Geometry: final body of the model. Coordinates: model frame, mm. Face numbers are marked on the shaded views. A direction names the side the tool comes from. Give positions to 0.01 mm unless a question says otherwise; leave off trailing zeros. Order: outer loops, then holes, each group sorted by start corner. A loop starts at its lowest first (then second) coordinate and runs counter-clockwise, first axis right, second up. Notation, with made-up numbers: (-2, 30) - (19, 30) arc R31 ccw to (19, 61) - close; hole circle Ø8 at (21.25, 82.5). An arc over 180 degrees is marked (long way). Use one line per item in the form item = value.
from build123d import *

# Parameters (mm, degrees)
SKETCH_1_W      = 42.3
SKETCH_1_H      = 42.3
SKETCH_1_R      = 11
SKETCH_1_R_2    = 1.5
EXTRUDE_1_DEPTH = 4
SKETCH_2_W      = 38
SKETCH_2_H      = 62.3
SKETCH_2_R      = 1.5
EXTRUDE_2_DEPTH = 4
CHAMFER_1_SIZE  = 6


with BuildPart() as part:
    # 스케치1 → 보스-돌출1 (new body)
    with BuildSketch(Plane.XY):
        Rectangle(SKETCH_1_W, SKETCH_1_H)
        Circle(SKETCH_1_R, mode=Mode.SUBTRACT)
        with Locations((-15.5, 15.5)):
            Circle(SKETCH_1_R_2, mode=Mode.SUBTRACT)
        with Locations(Location((15.5, 15.5, 0), (0, 0, 180))):
            Circle(SKETCH_1_R_2, mode=Mode.SUBTRACT)
        with Locations((15.5, -15.5)):
            Circle(SKETCH_1_R_2, mode=Mode.SUBTRACT)
        with Locations(Location((-15.5, -15.5, 0), (0, 0, 180))):
            Circle(SKETCH_1_R_2, mode=Mode.SUBTRACT)
    extrude(amount=EXTRUDE_1_DEPTH)

    # 스케치2 → 보스-돌출2 (add)
    with BuildSketch(Plane(origin=(21.15, 0, 0), x_dir=(0, 0, -1), z_dir=(1, 0, 0))):
        with Locations((15, -10)):
            Rectangle(SKETCH_2_W, SKETCH_2_H)
        with Locations((5.5, -31.15)):
            Circle(SKETCH_2_R, mode=Mode.SUBTRACT)
        with Locations(Location((24.5, -31.15, 0), (0, 0, 180))):
            Circle(SKETCH_2_R, mode=Mode.SUBTRACT)
    extrude(amount=EXTRUDE_2_DEPTH)

    # 모따기1
    chamfer_1_edges = [part.edges().sort_by_distance(p)[0] for p in [
        (23.15, -41.15, 4),
        (23.15, -41.15, -34),
    ]]
    chamfer(chamfer_1_edges, length=CHAMFER_1_SIZE)


solid = part.part
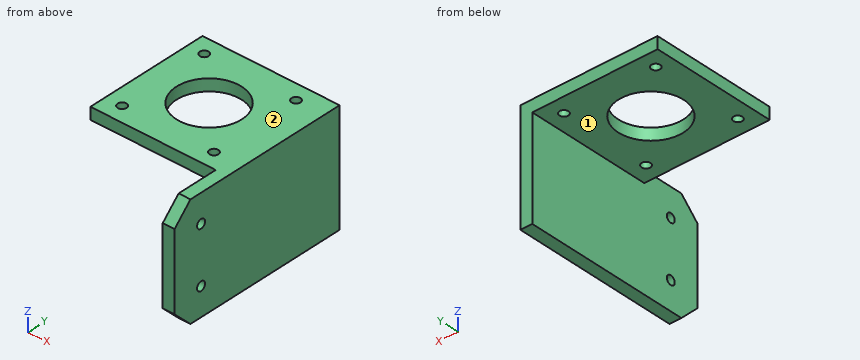
(1) Cut plane B-B on y = 0. Output: boundary loops of the cut face in (x, z), plus the area to 3 significant figures.
Computed values:
outline = (-21.15, 0) - (-11, 0) - (-11, 4) - (-21.15, 4) - close; (11, 0) - (21.15, 0) - (21.15, -34) - (25.15, -34) - (25.15, 4) - (11, 4) - close
area = 233 mm²
(2) Contact query for flat-ended pins moving along their axis: pin 1 Ø12 at (x, y) = (4, 6.5) entering from +Z; pin 2 Ø3 at (x, y) = (-15.5, 4.5) entering from -Z; pin 3 Ø4 at (y, z) = (-31.15, -24.5) entering from -X; pin 4 Ø3 at (x, z) = (9, 1.5) entering from -Y. Output: stop coordinate, or through.
Computed values:
pin_1 = 4
pin_2 = 0
pin_3 = 21.15
pin_4 = -21.15
(3) Cut plane A-A on x = 15.5. Output: boundary loops of the cut face in (y, z), plus the area to 3 significant figures.
Computed values:
outline = (-21.15, 0) - (-17, 0) - (-17, 4) - (-21.15, 4) - close; (-14, 0) - (14, 0) - (14, 4) - (-14, 4) - close; (17, 0) - (21.15, 0) - (21.15, 4) - (17, 4) - close
area = 145 mm²
(4) Reachability of the marked faces 1 and 2 from +Z, -Z, +X, -X, +Y, -Y: full face, straight path, thin tool, end or side. Return the list, or none.
Computed values:
face_1 = -Z, -X, +Y, -Y
face_2 = +Z, +X, -X, +Y, -Y
(5) Ray query, line 1 along Y through (x, z) = (-15.5, 2.1); line 2 along Y through (x, z) = (0, 2.75); line 3 along Y through (x, z) = (-15, 1). Return the intervals inside material, ascending.
Computed values:
line_1 = -21.15 to -17, -14 to 14, 17 to 21.15
line_2 = -21.15 to -11, 11 to 21.15
line_3 = -21.15 to -16.91, -14.09 to 14.09, 16.91 to 21.15
(6) Cut plane C-C on x = 0. Output: boundary loops of the cut face in (y, z), plus the area to 3 significant figures.
Computed values:
outline = (-21.15, 0) - (-11, 0) - (-11, 4) - (-21.15, 4) - close; (11, 0) - (21.15, 0) - (21.15, 4) - (11, 4) - close
area = 81.2 mm²
(7) Cut plane D-D on z = -5.5. Output: boundary loops of the cut face in (x, y).
Computed values:
outline = (21.15, -41.15) - (25.15, -41.15) - (25.15, -32.65) - (21.15, -32.65) - close; (21.15, -29.65) - (25.15, -29.65) - (25.15, 21.15) - (21.15, 21.15) - close
